```python
from build123d import *

# Parameters (mm, degrees)
SKETCH_1_R               = 20
EXTRUDE_1_DEPTH          = 20
EXTRUDE_2_DEPTH          = 20
PATTERN_CIRCULAR_1_COUNT = 8
CUT_EXTRUDE_1_DEPTH      = 34
SKETCH_5_R               = 12.5
CUT_EXTRUDE_2_DEPTH      = 4


with BuildPart() as part:
    # Sketch 1 → Extrude 1 (new body)
    with BuildSketch(Plane(origin=(0, 0, 0), x_dir=(1, 0, 0), z_dir=(0, 1, 0))):
        Circle(SKETCH_1_R)
    extrude(amount=EXTRUDE_1_DEPTH)

    # Sketch 3 → Extrude 2 (add)
    with BuildSketch(Plane(origin=(0, 20, 0), x_dir=(1, 0, 0), z_dir=(0, 1, 0))):
        with BuildLine():
            Line((-2, -20.90454496), (-2, 20.90454496))
            ThreePointArc((-2, 20.90454496), (0, 21), (2, 20.90454496))
            Line((2, 20.90454496), (2, -20.90454496))
            ThreePointArc((2, -20.90454496), (0, -21), (-2, -20.90454496))
        make_face()
    extrude_2 = extrude(amount=-EXTRUDE_2_DEPTH)

    # Pattern Circular 1: Extrude 2 ×8 about axis
    pattern_circular_1_axis = Axis((0, 0, 0), (0, 1, 0))
    for i in range(1, PATTERN_CIRCULAR_1_COUNT):
        add(extrude_2.rotate(pattern_circular_1_axis, i * 360 / PATTERN_CIRCULAR_1_COUNT))

    # Sketch 2 → Cut-Extrude 1 (cut, symmetric)
    with BuildSketch(Plane.XY):
        Polygon((-21.218882006, 2), (25.661502265, 14.561561106), (25.661502265, 41.51194957), (-21.218882006, 43.85785004), align=None)
    extrude(amount=CUT_EXTRUDE_1_DEPTH, both=True, mode=Mode.SUBTRACT)

    # Sketch 5 → Cut-Extrude 2 (cut)
    with BuildSketch(Plane(origin=(-1.921395574, 7.170745905, 0), x_dir=(0.965925826, 0.258819045, 0), z_dir=(-0.258819045, 0.965925826, 0))):
        with Locations((1.989175071, 0)):
            Circle(SKETCH_5_R)
    extrude(amount=-CUT_EXTRUDE_2_DEPTH, mode=Mode.SUBTRACT)


solid = part.part
```
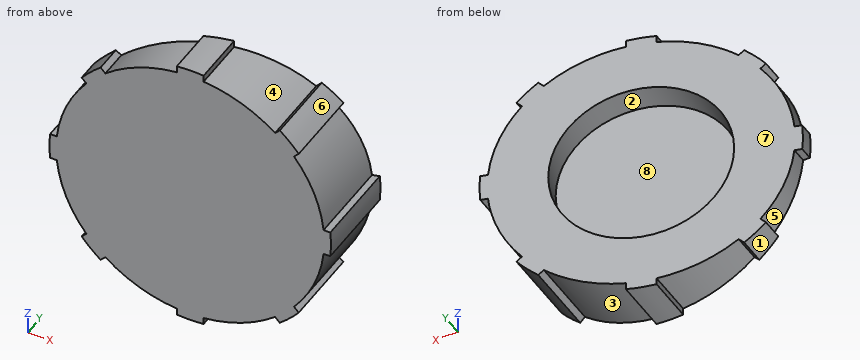
Geometry check sheet. Reference: the model listing, model coordinates, mm. Face numbers are marked on the shaded views. A direction names the side the tool comes from. Coordinates: 2 decimals unless noted, no trailing zeros. Loops run counter-clockwise (first coordinate to the right, second up) from the corner with the lowest first, then second, coordinate; pieces in that order, holes last. Notation, with made-up numbers: (59, -16.5) -> (69, -16.5) arc R9 ccw to (69, -0.5) -> close; hole circle Ø5 at (-14, 80.25). An arc over 180 degrees is marked (long way). Put each result on its own line as item: value.
1) Cross-section at A-A on z = -11. Record the boundary of the cut face in (x, y).
Result set:
outline: (-16.7, 0) -> (16.7, 0) -> (16.7, 12.16) -> (5.73, 9.22) -> (6.77, 5.36) -> (-4.7, 2.29) -> (-5.73, 6.15) -> (-16.7, 3.21) -> close
2) Thickness scan on line 1 (Y direction, x = 18, z = -0.5); line 2 (Z direction, x = 10, y = 9.75); line 3 (Y direction, x = -16.5, z = -8). Record the ranges inside material, lowest first.
Result set:
line 1: y = 0 to 12.51
line 2: z = -17.32 to -7.23, 7.23 to 17.32
line 3: y = 0 to 3.26
3) Cross-section at D-D on x = 18. Record the boundary of the cut face in (y, z), plus the area to 3 significant figures.
Result set:
outline: (0, -8.72) -> (12.51, -8.72) -> (12.51, 8.72) -> (0, 8.72) -> close
area: 218 mm^2
4) Cross-section at B-B on x = -14. Record the boundary of the cut face in (y, z), plus the area to 3 significant figures.
Result set:
outline: (0, -15.65) -> (3.93, -15.65) -> (3.93, 15.65) -> (0, 15.65) -> close
area: 123 mm^2
5) Cross-section at C-C on z = 12. Record the boundary of the cut face in (x, y), plus the area to 3 significant figures.
Result set:
outline: (-16, 0) -> (16, 0) -> (16, 11.97) -> (3.38, 8.59) -> (4.42, 4.73) -> (-2.35, 2.92) -> (-3.38, 6.78) -> (-16, 3.4) -> close
area: 218 mm^2
6) Gauge pin test, flat ends, axial feed: pin 1 Ø3 at (y, z) = (2, 4) entering from +X; pin 2 Ø3 at (y, z) = (4.5, -9.5) entering from +X; pin 3 Ø12 at (x, z) = (7.5, 16) entering from +Y; pin 4 Ø6 at (x, y) = (-11.5, 8.5) entering from -Z. Record the tip position at first contact, or that the pin passes through.
Result set:
pin 1: stops at x = 19.84
pin 2: stops at x = 18.33
pin 3: stops at y = 11.3
pin 4: passes through
7) Tool access check on the marked faces 1, 2, 3, 4 and 5. Record the directions out of +Z, -Z, +X, -X, +Y, -Y that give a thin tool (end or side, any length) a straight path to the whole face; none if there is none.
Result set:
face 1: -Z, -X, +Y, -Y
face 2: none
face 3: -Z, +Y, -Y
face 4: +Z, +Y, -Y
face 5: -X, +Y, -Y
8) Release check for a two-part mould opening along X. For the marked faces 6, 7 and 8 record: released by +X, released by -X, zero draft, split by the parting line, or undercut.
Result set:
face 6: released by +X
face 7: released by -X
face 8: undercut
